The listing builds one solid part. Answer for the finished solid, in the listing's coordinates (mm). A direction names the side the tool comes from. Give positions to 0.01 mm unless a question says otherwise; leave off trailing zeros. Write each loop counter-clockwise with the first axis right and the second up, starting at its lowest first coordinate (ties: lowest second). Pieces come first, ordered by that corner, then holes. Notation, with made-up numbers: (32.25, 56) - (83.25, 56) arc R27 ccw to (83.25, 76) - close; hole circle Ø11 at (44.25, 21). An arc over 180 degrees is marked (long way). Return JSON: item names as keys, results as strings.
from build123d import *

# Parameters (mm, degrees)
SKETCH6_R           = 25.4
BOSS_EXTRUDE2_DEPTH = 25.4
SKETCH7_R           = 22.86
CUT_EXTRUDE1_DEPTH  = 91.807220253
SKETCH8_R           = 27.94
CUT_EXTRUDE2_DEPTH  = 31.75
FILLET1_R           = 0.635


with BuildPart() as part:
    # Sketch5 → Revolve1 (revolve)
    with BuildSketch(Plane.XY, mode=Mode.PRIVATE) as revolve1_sk:
        Polygon((0, 0), (0, 50.8), (-34.925, 50.8), (-26.0604, 0), align=None)
    revolve(revolve1_sk.sketch.rotate(Axis((0, 0, 0), (0, 1, 0)), 270), axis=Axis((0, 0, 0), (0, 1, 0)))

    # Sketch6 → Boss-Extrude2 (add)
    with BuildSketch(Plane.XZ):
        with Locations(Location((0, 0, 0), (0, 0, 270))):
            Circle(SKETCH6_R)
    extrude(amount=BOSS_EXTRUDE2_DEPTH)

    # Sketch7 → Cut-Extrude1 (cut, through all)
    with BuildSketch(Plane.XZ.offset(25.4)):
        with Locations(Location((0, 0, 0), (0, 0, 270))):
            Circle(SKETCH7_R)
    extrude(amount=-CUT_EXTRUDE1_DEPTH, mode=Mode.SUBTRACT)

    # Sketch8 → Cut-Extrude2 (cut)
    with BuildSketch(Plane(origin=(0, 50.8, 0), x_dir=(1, 0, 0), z_dir=(0, 1, 0))):
        with Locations(Location((0, 0, 0), (0, 0, 270))):
            Circle(SKETCH8_R)
    extrude(amount=-CUT_EXTRUDE2_DEPTH, mode=Mode.SUBTRACT)

    # Fillet1
    fillet1_edges = [part.edges().sort_by_distance(p)[0] for p in [
        (0, 19.05, -27.94),
        (0, 19.05, 22.86),
    ]]
    fillet(fillet1_edges, radius=FILLET1_R)


solid = part.part
Item 1: For faces 5 (the face through (25, 0, -6)), 6 (the face through (10, -25.4, 21)), determine the directions among +Z, -Z, +X, -X, +Y, -Y from which every point of the face is accessible in a straight line to the end or side of a thin tool.
Answer below:
{"face 5": "-Y", "face 6": "+Z, -Z, +X, -X, -Y"}
Item 2: The mould has two halves that part along X. Classify faces 1 (the face through (-15.456, -12.522, 20.157)), 2 (the face through (20.4, 19.05, 12)), 3 (the face through (-23.4, 50.8, -15.7)), 4 (the face through (27.7, 35.46, -3.64)): +X half, -X half, draft (parallel to the pull), parting line (faces both ways), or undercut.
Answer below:
{"face 1": "parting line", "face 2": "undercut", "face 3": "draft", "face 4": "undercut"}
Item 3: A cutting plane is placed at C-C on y = -6. Determine the outline of the cut face in (x, z).
Answer below:
{"outline": "circle Ø50.8 at (0, 0); hole circle Ø45.72 at (0, 0)"}
Item 4: A cutting plane is placed at B-B on x = 0. Determine the outline of the cut face in (y, z) (3 decimals), then the cut area to 3 significant figures.
Answer below:
{"outline": "(-25.4, -25.4) - (0, -25.4) - (0, -26.06) - (50.8, -34.925) - (50.8, -27.94) - (19.685, -27.94) arc R0.635 cw to (19.05, -27.305) - (19.05, -23.495) arc R0.635 ccw to (18.415, -22.86) - (-25.4, -22.86) - close; (-25.4, 22.86) - (18.415, 22.86) arc R0.635 ccw to (19.05, 23.495) - (19.05, 27.305) arc R0.635 cw to (19.685, 27.94) - (50.8, 27.94) - (50.8, 34.925) - (0, 26.06) - (0, 25.4) - (-25.4, 25.4) - close", "area": "582 mm²"}
Item 5: Consider L1, parallel to X at y = -4, z = 0; L2, parallel to Z at x = -19, y = 37; L3, parallel to Z at x = -13, y = 17.5. Determine where each line is inside the solid, lowest interval first.
Answer below:
{"L1": "x = -25.4 to -22.86, 22.86 to 25.4", "L2": "z = -26.39 to -20.49, 20.49 to 26.39", "L3": "z = -26.05 to -18.8, 18.8 to 26.05"}
Item 6: A cutting plane is placed at D-D on y = 4. Determine the outline of the cut face in (x, z), then the cut area to 3 significant figures.
Answer below:
{"outline": "circle Ø53.52 at (0, 0); hole circle Ø45.72 at (0, 0)", "area": "608 mm²"}
Item 7: A cutting plane is placed at A-A on z = 0. Determine the outline of the cut face in (x, y) (3 decimals), then the cut area to 3 significant figures.
Answer below:
{"outline": "(-34.925, 50.8) - (-26.06, 0) - (-25.4, 0) - (-25.4, -25.4) - (-22.86, -25.4) - (-22.86, 18.415) arc R0.635 ccw to (-23.495, 19.05) - (-27.305, 19.05) arc R0.635 cw to (-27.94, 19.685) - (-27.94, 50.8) - close; (22.86, -25.4) - (25.4, -25.4) - (25.4, 0) - (26.06, 0) - (34.925, 50.8) - (27.94, 50.8) - (27.94, 19.685) arc R0.635 cw to (27.305, 19.05) - (23.495, 19.05) arc R0.635 ccw to (22.86, 18.415) - close", "area": "582 mm²"}
Item 8: Flat-ended cylindrical pins translate along their axes: P1, Ø1.5, axis at y = -6.5, z = 13, coming from the -X side; P2, Ø12, axis at y = 23.5, z = 6, coming from the +X side; P3, Ø6, axis at y = 32, z = 24, coming from the -X side. Find the tip coordinate at first contact, or state that the pin passes through.
Answer below:
{"P1": "stops at x = -22.25", "P2": "stops at x = 30.92", "P3": "stops at x = -23.76"}
